Autodesk Inventor part; units mm, degrees
ref_plane "YZ Plane" through (0, 0, 0) normal (1, 0, 0) x (0, 1, 0)
ref_plane "XZ Plane" through (0, 0, 0) normal (0, 1, 0) x (-1, 0, 0)
ref_plane "XY Plane" through (0, 0, 0) normal (0, 0, 1) x (1, 0, 0)
sketch "Sketch1" plane through (0, 0, 0) normal (0, 1, 0) x (-1, 0, 0)
  line L0 (7, 7) -> (-7, 7)
  line L1 (-7, 7) -> (-7, -7)
  line L2 (-7, -7) -> (7, -7)
  line L3 (7, -7) -> (7, 7)
  line L4 (7, 7) -> (-7, -7) construction
  line L5 (-7, 7) -> (7, -7) construction
  line L6 (6, 6) -> (-6, 6)
  line L7 (-6, 6) -> (-6, -6)
  line L8 (-6, -6) -> (6, -6)
  line L9 (6, -6) -> (6, 6)
  point P0 (0, 0)
  dimension "d0" = 14
  dimension "d1" = 14
  dimension "d2" = 1
extrude "Extrusion1" add sketch "Sketch1" along normal blind 5
sketch "Sketch2" plane through (0, 5, 0) normal (0, 1, 0) x (1, 0, 0)
  line L0 (-7, -7) -> (7, -7)
  line L1 (3, -7) -> (7, -3)
  line L2 (7, -7) -> (7, 7)
  line L3 (-7, 7) -> (-7, -7)
  line L4 (-7, 3) -> (-3, 7)
  line L5 (7, 7) -> (-7, 7)
  point P0 (0, 0)
  dimension "d5" = 4
  dimension "d6" = 4
  dimension "d7" = 4
  dimension "d8" = 4
extrude "Extrusion2" add sketch "Sketch2" along normal mid plane 10 contours L1 L2 L0 | L3 L5 L4
sketch "Sketch3" plane through (0, 0, 0) normal (0, -1, 0) x (1, 0, 0)
  line L0 (7, -7) -> (-7, -7)
  line L1 (7, 7) -> (7, -7)
  line L2 (-7, 7) -> (7, 7)
  line L3 (-7, -7) -> (-7, 7)
  line L4 (-4, -6) -> (-6, -4)
  line L5 (-6, 6) -> (-6, -4)
  line L6 (4, 6) -> (-6, 6)
  line L7 (4, 6) -> (6, 4)
  line L8 (6, -6) -> (6, 4)
  line L9 (-4, -6) -> (6, -6)
  point P0 (0, 0)
extrude "Extrusion3" add sketch "Sketch3" against normal blind 1 contours L0 L3 L2 L1 | L4 L5 L6 L7 L8 L9
sketch "Sketch4" plane through (0, 1, 0) normal (0, 1, 0) x (1, 0, 0)
  circle A0 centre (-4, -4) radius 0.9814
  circle A1 centre (4, 4) radius 0.9814
  line L0 (-6, -6) -> (-6, 4)
  line L1 (4, -6) -> (-6, -6)
  line L2 (-4, 6) -> (6, 6)
  line L3 (6, 6) -> (6, -4)
  point P0 (0, 0)
  dimension "d15" = 2
  dimension "d16" = 2
  dimension "d17" = 2
  dimension "d18" = 2
extrude "Extrusion4" add sketch "Sketch4" along normal blind 9
sketch "Sketch5" plane through (-3, 5, -7) normal (0.7071, 0, 0.7071) x (0.7071, 0, -0.7071)
  line L0 (-2.8284, -5) -> (-2.8284, 5)
  circle A0 centre (-2.8284, 3.1472) radius 0.25
  dimension "d19" = 0.5
extrude "Extrusion5" cut sketch "Sketch5" along normal blind 14.75 and the other way blind 0.75
properties part number "disk holder" material "ABS Plastic"
CAD build for the part. Positions are in the model's coordinates, mm. A direction names the side the tool comes from. Coordinates: 2 decimals unless noted, no trailing zeros. Loops run counter-clockwise (first coordinate to the right, second up) from the corner with the lowest first, then second, coordinate; pieces in that order, holes last. Notation, with made-up numbers: (75, 50) - (129, 50) arc R16 ccw to (129, 69) - close; hole circle Ø4 at (-30.5, 20.25). An arc over 180 degrees is marked (long way). Use one line per item in the form item = value. Start each with the question number.
1) Drill centre lines: L1, parallel to Z at x = 2, y = 1.25; L2, parallel to X at y = 6, z = 4. Where is each one in solid material? Low to high. Write a range as from..to.
2) Band-saw the part on C-C (y = 9.5). Give the cut face in (x, z).
3) Band-saw the part on D-D (z = -0.5). Give the cut face in (x, y), and give its area (3 significant figures).
4) Two-plate mould, pull along X, no slides. Class faces 3 (the face through (-4, 10, 4)), 4 (the face through (-1, 3, 6)), 5 (the face through (7, 4, 2)): +X half, -X half, draft (parallel to the pull), parting line (faces both ways), or undercut.
5) Band-saw the part on B-B (x = -0.25). Give the cut face in (y, z), and give its area (3 significant figures).
6) Flat gauge pins, fed straight in: pin 1 (6 mm diameter, centred on x = 2, z = 2.5, fed in from +Y); pin 2 (1 mm diameter, centred on x = -4, y = 6, fed in from +Z). Where does each tip first touch, or does it go through?
7) Band-saw the part on A-A (y = 4.75). Give the cut face in (x, z).
8) Tool access for faces 1 (the face through (6, 3, -1)), 2 (the face through (-5.5, 10, -5.5)): list every direction of +Z, -Z, +X, -X, +Y, -Y with a clear straight run to the whole face (end or side of a thin tool).
Check values:
q1.L1 = -7..-6, 6..7
q1.L2 = -4.98..-3.02, 6..7
q2.outline = (-7, -7) - (-3, -7) - (-7, -3) - close; circle Ø1.96 at (-4, 4); (3, 7) - (7, 3) - (7, 7) - close; circle Ø1.96 at (4, -4)
q3.outline = (-7, 0) - (7, 0) - (7, 5) - (6, 5) - (6, 1) - (-6, 1) - (-6, 5) - (-7, 5) - close
q3.area = 22.0 mm2
q4.face_3 = draft
q4.face_4 = undercut
q4.face_5 = +X half
q5.outline = (0, -7) - (5, -7) - (5, -6) - (1, -6) - (1, 6) - (5, 6) - (5, 7) - (0, 7) - close
q5.area = 22.0 mm2
q6.pin_1 = 1
q6.pin_2 = 4.98
q7.outline = (-7, -7) - (7, -7) - (7, 7) - (-7, 7) - close; circle Ø1.96 at (-4, 4); circle Ø1.96 at (4, -4); hole (-6, -4) - (-4, -6) - (6, -6) - (6, 4) - (4, 6) - (-6, 6) - close
q8.face_1 = +Y
q8.face_2 = +Z, -Z, +X, -X, +Y
